Check sheet for the modelled part. Datum: model origin and axes. Units: mm. A direction names the side the tool comes from. Give positions to 0.01 mm unless a question says otherwise; leave off trailing zeros. Write each loop counter-clockwise with the first axis right and the second up, starting at its lowest first coordinate (ties: lowest second). Pieces come first, ordered by that corner, then holes.
from build123d import *

# Parameters (mm, degrees)
SKETCH_1_W          = 20
SKETCH_1_H          = 30
EXTRUDE_1_DEPTH     = 18
CUT_EXTRUDE_4_DEPTH = 41.298883359


with BuildPart() as part:
    # Эскиз1 → Вытянуть1 (new body)
    with BuildSketch(Plane(origin=(0, 0, 0), x_dir=(0, 0, -1), z_dir=(1, 0, 0))):
        with Locations((-10, -6.749432462)):
            Rectangle(SKETCH_1_W, SKETCH_1_H)
    extrude(amount=EXTRUDE_1_DEPTH)

    # Эскиз2 → Вырез-Вытянуть4 (cut, through all)
    with BuildSketch(Plane(origin=(0, 8.250567538, 0), x_dir=(1, 0, 0), z_dir=(0, 1, 0))):
        with BuildLine():
            Line((-0.004897471, 0.146832679), (18, 0.146832679))
            Line((18, 0.146832679), (18, -0.382236535))
            ThreePointArc((18, -0.382236535), (17.0627417, -2.644978234), (14.8, -3.582236535))
            Line((14.8, -3.582236535), (3.195102529, -3.582236535))
            ThreePointArc((3.195102529, -3.582236535), (0.932360829, -2.644978234), (-0.004897471, -0.382236535))
            Line((-0.004897471, -0.382236535), (-0.004897471, 0.146832679))
        make_face()
    extrude(amount=-CUT_EXTRUDE_4_DEPTH, mode=Mode.SUBTRACT)


solid = part.part
1) Sectioned sample at D-D on x = 16. Record the boundary of the cut face in (y, z), then the cut area to 3 significant figures.
2) Scan lines: L1, parallel to Z at x = 4.5, y = -11; L2, parallel to Z at x = 15.75, y = -5.25; L3, parallel to X at y = -4.5, z = 1.75. Record each from-to range of solid material in increasing order.
3) Draft check along X on faces 1 (the flat face through (0, -7, 10)), 2 (the cylindrical face through (1.02, -6.54, 2.73)), 3 (the flat face through (18, -7, 10)), 4 (the flat face through (9, -21.749, 13)). Enter one of: +X half, -X half, draft (parallel to the pull), parting line (faces both ways), or undercut.
4) Sectioned sample at B-B on y = -19. Record the boundary of the cut face in (x, z), then the cut area to 3 significant figures.
5) Sectioned sample at C-C on x = 5.5. Record the boundary of the cut face in (y, z).
6) Access from +Z, -Z, +X, -X, +Y, -Y to the whole of each face (thin tool, end or side, straight path). Record for faces 5 (the cylindrical face through (17.09, -6.54, 2.62)), 6 (the flat face through (9, -7, 20)).
7) Gauge pin test, flat end, axial feed: pin 1 (6 mm diameter, centred on x = 11.5, y = -3.5, fed in from -Z). Record the tip position at first contact, or that the pin passes through.
8) Sectioned sample at A-A on z = 2.25. Record the boundary of the cut face in (x, y).
Answers below:
1. outline: (-21.75, 3.35) - (8.25, 3.35) - (8.25, 20) - (-21.75, 20) - close
1. area: 500 mm2
2. L1: z = 3.58 to 20
2. L2: z = 3.44 to 20
2. L3: x = 0 to 0.3, 17.69 to 18
3. face 1: -X half
3. face 2: undercut
3. face 3: +X half
3. face 4: draft
4. outline: (0, 0.56) arc R3.2 cw to (3.2, 3.58) - (14.8, 3.58) arc R3.2 cw to (18, 0.38) - (18, 20) - (0, 20) - close
4. area: 300 mm2
5. outline: (-21.75, 3.58) - (8.25, 3.58) - (8.25, 20) - (-21.75, 20) - close
6. face 5: -Z, +Y, -Y
6. face 6: +Z, +X, -X, +Y, -Y
7. pin 1: stops at z = 3.58
8. outline: (0, -21.75) - (0.6, -21.75) - (0.6, 8.25) - (0, 8.25) - close; (17.4, -21.75) - (18, -21.75) - (18, 8.25) - (17.4, 8.25) - close
